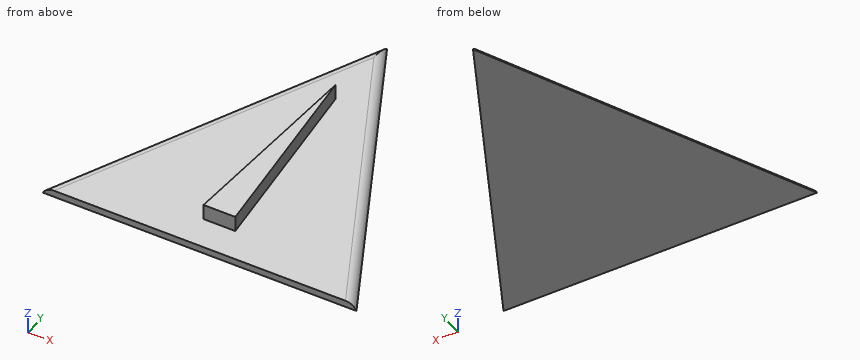
```python
from build123d import *

# Parameters (mm, degrees)
F1_DEPTH    = 3.302
F2_T1_DEPTH = 194.5409515442
F2_T3_DEPTH = 194.4495264649
F4_DEPTH    = 7.62


# Not quite as in the source:
# - a fillet or chamfer that OpenCascade refuses, or shapes differently, is made with other operations: its cross-section is extruded or revolved along the edge and cut away or added


with BuildPart() as f1:
    # F0 (on Top) → F1 (new body)
    with BuildSketch(Plane.XY):
        Polygon((75.576454401, -75.9910270572), (0, 77.0177915692), (-75.7826715708, -75.9910270572), align=None)
    extrude(amount=F1_DEPTH)

    # F2: fillet of radius 5.08 on 2 edges, made by hand

    # F2_s2 → F2_t1 (cut)
    with BuildSketch(Plane(origin=(35.9116375184, 72.5073043447, 0), x_dir=(0, 0, 1), z_dir=(-0.4438288555, -0.8961115706, 0))):
        with BuildLine():
            ThreePointArc((0, 34.1827182836), (2.3956458882, 32.3200753886), (3.302, 29.4240298088))
            Line((3.302, 29.4240298088), (3.302, 34.1827182836))
            Line((3.302, 34.1827182836), (0, 34.1827182836))
        make_face()
    extrude(amount=F2_T1_DEPTH, mode=Mode.SUBTRACT)

    # F2_s4 → F2_t3 (cut)
    with BuildSketch(Plane(origin=(50.2640998489, -101.7625211206, 0), x_dir=(0, 0, 1), z_dir=(-0.4428582479, 0.8965916418, 0))):
        with BuildLine():
            ThreePointArc((0, 34.1079642346), (2.3956458882, 32.2453213396), (3.302, 29.3492757599))
            Line((3.302, 29.3492757599), (3.302, 34.1079642346))
            Line((3.302, 34.1079642346), (0, 34.1079642346))
        make_face()
    extrude(amount=F2_T3_DEPTH, mode=Mode.SUBTRACT)

    # F3 (on face) → F4 (join)
    with BuildSketch(Plane.XY.offset(3.302)):
        Polygon((7.7744186856, -60.2337494493), (0, 34.9251665175), (-7.5671025552, -60.2337494493), align=None)
    extrude(amount=F4_DEPTH)


solid = f1.part
```
Work out the finished part from the listing and answer in its coordinate system (mm). Give positions to 0.01 mm unless a question says otherwise; leave off trailing zeros. Loops run counter-clockwise (first coordinate to the right, second up) from the corner with the lowest first, then second, coordinate; pieces in that order, holes last. Notation, with made-up numbers: (57.25, 70.25) -> (106.25, 70.25) arc R22 ccw to (106.25, 91.25) -> close; hole circle Ø8 at (76, 10.25). An arc over 180 degrees is marked (long way). Write item = value, one per line. Start each with the question number.
(1) Find section A-A on z = 5.5. Give the vertices of the cut face in (x, y).
(2) Given pin 1 Ø8 at (x, y) = (31.5, 22) entering from +Z; pin 2 Ø5 at (y, z) = (50, 6) entering from +X; pin 3 Ø4 at (x, z) = (0, 6.5) entering from -Y, each flat-ended and moving along its own axis, determine where each tip first touches the part or whether it passes through.
(3) Find the intervals of material crossed by probe 1 along Z at (x, y) = (18.5, -61.5); probe 2 along X at (y, z) = (-46, 9.75); probe 3 along Y at (x, z) = (-32.5, 1.5), in increasing order. Write a range as from..to.
From the geometry:
q1.outline = (-7.57, -60.23) -> (7.77, -60.23) -> (0, 34.93) -> close
q2.pin_1 = 0.3
q2.pin_2 = through
q2.pin_3 = -60.23
q3.probe_1 = 0..3.3
q3.probe_2 = -6.44..6.61
q3.probe_3 = -75.99..9.42
